For this review, take the finished solid that the model builds, in its own axes (mm). A direction names the side the tool comes from. Round coordinates to 2 decimals unless told otherwise and drop trailing zeros. Order: outer loops, then holes, each group sorted by start corner. A loop starts at its lowest first (then second) coordinate and runs counter-clockwise, first axis right, second up. Notation, with made-up numbers: (35.25, 86) -> (78.25, 86) arc R13 cw to (78.25, 94) -> close; hole circle Ø6 at (85, 14.25). An arc over 180 degrees is marked (long way). Use a Markdown table: item, result. Add a question column.
1) Clearance check with flat-ended pins moving along their axes: P1, Ø3, axis at y = -11.5, z = 10.5, coming from the +X side; P2, Ø3, axis at y = -13.5, z = 4, coming from the +X side; P3, Ø4, axis at y = -14.5, z = 8.5, coming from the -X side; P4, Ø3, axis at x = 6.5, y = -12, coming from the +Z side. State where each tip first meets the part, or that it passes through.
2) Consider section B-B (y = -14.5). Give the number of separate pieces and of enclosed holes in the cut face, plus the area to 3 significant figures.
3) Consider section A-A (z = 7.25). State the section outline as (x, y) points, plus the area to 3 significant figures.
4) Consider section D-D (z = 5). State the section outline as (x, y) points, plus the area to 3 significant figures.
5) Wall thickness on line 1 along X through (y, z) = (-12, 5.5); line 2 along Z through (x, y) = (3.5, -11.25); line 3 along Z through (x, y) = (-2, -15.5): over which ranges is each line inside the solid? List them lowest first. Write a range as [from, to].
6) Draft analysis for pull direction Z (two halves, no side actions). For faces 1 (the face through (4.717, -11, 8)), 2 (the face through (10.95, -12.46, 5.44)), 3 (the face through (2, -11.625, 8)), state which applies: pulls with the +Z half, pulls with the -Z half, needs draft (parallel to the pull), parting line crosses it, or undercut.
7) Consider section C-C (x = 0.25). State the section outline as (y, z) points, plus the area to 3 significant figures.
8) Machinability: for faces 4 (the face through (-3, -12, 6.35)), 5 (the face through (2, -11.625, 11)), 6 (the face through (1.656, -15.016, 11.611)), which of the approach directions +Z, -Z, +X, -X, +Y, -Y give a long, thin tool a straight path to every point of the face, cutting with its end or side? Answer none if there is none.
```python
from build123d import *

# Parameters (mm, degrees)
F0_W        = 20.6375
F0_H        = 7
F1_DEPTH    = 6.35
F2_R        = 2.794
F3_DEPTH    = 8
F4_R        = 3.17499
F5_W        = 6.0368906707
F5_H        = 7
F6_DEPTH    = 6.35
F7_T1_DEPTH = 23.8168906707
F8_W        = 2
F8_H        = 5
F9_DEPTH    = 6.35
F10_W       = 1.5076477192
F10_H       = 2
F10_W_2     = 1.4923522808
F10_W_3     = 2
F10_H_2     = 1.5520717202
F11_DEPTH   = 6.35


# Not quite as in the source:
# - a fillet or chamfer that OpenCascade refuses, or shapes differently, is made with other operations: its cross-section is extruded or revolved along the edge and cut away or added
# - a fillet or chamfer is up to 0.001 mm smaller than in the source, because OpenCascade refuses the exact size


with BuildPart() as f1:
    # F0 (on Top) → F1 (new body)
    with BuildSketch(Plane.XY):
        with Locations((1.5829298645, -12.5110630834)):
            Rectangle(F0_W, F0_H)
    extrude(amount=F1_DEPTH)

    # F2 (on face) → F3 (cut)
    with BuildSketch(Plane.XZ.offset(16.0110630834)):
        with Locations((-5.4325845507, 3.1855095279)):
            Circle(F2_R)
        with Locations((1.5883980845, 3.2361580911)):
            Circle(F2_R)
        with Locations((8.5595190756, 3.1868351264)):
            Circle(F2_R)
    extrude(amount=-F3_DEPTH, mode=Mode.SUBTRACT)

    # F4 (radius 3.175 in the source; OpenCascade refuses exactly that, so slightly less here)
    f4_edges = [f1.edges().sort_by_distance(p)[0] for p in [
        (11.90168, -12.511063, 6.35),
        (11.90168, -12.511063, 0),
        (-8.73582, -12.511063, 6.35),
        (-8.73582, -12.511063, 0),
    ]]
    fillet(f4_edges, radius=F4_R)

    # F5 (on face) → F6 (join)
    with BuildSketch(Plane.XY.offset(6.35)):
        with Locations((1.6981104854, -12.5110630834)):
            Rectangle(F5_W, F5_H)
    extrude(amount=F6_DEPTH)

    # F7: fillet of radius 3.556 on 2 edges, made by hand

    # F7_s2 → F7_t1 (cut)
    with BuildSketch(Plane.YZ.offset(-10.2103348499)):
        with BuildLine():
            ThreePointArc((-16.0110630834, 9.144), (-14.9695347973, 11.6584717139), (-12.4550630834, 12.7))
            Line((-12.4550630834, 12.7), (-16.0110630834, 12.7))
            Line((-16.0110630834, 12.7), (-16.0110630834, 9.144))
        make_face()
        with BuildLine():
            ThreePointArc((-9.0110630834, 9.144), (-10.0525913695, 11.6584717139), (-12.5670630834, 12.7))
            Line((-12.5670630834, 12.7), (-9.0110630834, 12.7))
            Line((-9.0110630834, 12.7), (-9.0110630834, 9.144))
        make_face()
    extrude(amount=F7_T1_DEPTH, mode=Mode.SUBTRACT)

    # F8 (on face) → F9 (cut)
    with BuildSketch(Plane(origin=(-1.3203348499, 0, 0), x_dir=(0, -1, 0), z_dir=(-1, 0, 0))):
        with Locations((12.6245897673, 9.4653457722)):
            Rectangle(F8_W, F8_H)
    extrude(amount=-F9_DEPTH, mode=Mode.SUBTRACT)

    # F10 (on face) → F11 (cut)
    with BuildSketch(Plane.YZ.offset(4.7165558208)):
        with Locations((-14.3784136269, 9.5174174924)):
            Rectangle(F10_W, F10_H)
        with Locations((-10.8784136269, 9.5174174924)):
            Rectangle(F10_W_2, F10_H)
        with Locations((-12.6245897673, 7.7413816323)):
            Rectangle(F10_W_3, F10_H_2)
    extrude(amount=-F11_DEPTH, mode=Mode.SUBTRACT)


solid = f1.part
```
Results list:
| question | item | result |
|---|---|---|
| 1 | P1 | x = 4.72 |
| 1 | P2 | x = 11.9 |
| 1 | P3 | x = -1.32 |
| 1 | P4 | z = 6.35 |
| 2 | separate pieces | 2 |
| 2 | enclosed holes | 3 |
| 2 | area | 71.2 mm2 |
| 3 | outline | (-1.32, -16.01) -> (4.72, -16.01) -> (4.72, -13.62) -> (-1.32, -13.62) -> close; (-1.32, -11.62) -> (4.72, -11.62) -> (4.72, -9.01) -> (-1.32, -9.01) -> close |
| 3 | area | 30.2 mm2 |
| 4 | outline | (-8.16, -16.01) -> (-7.56, -16.01) -> (-7.56, -9.01) -> (-8.16, -9.01) -> close; (-3.31, -16.01) -> (-0.58, -16.01) -> (-0.58, -9.01) -> (-3.31, -9.01) -> close; (3.76, -16.01) -> (6.43, -16.01) -> (6.43, -9.01) -> (3.76, -9.01) -> close; (10.69, -16.01) -> (11.32, -16.01) -> (11.32, -9.01) -> (10.69, -9.01) -> close |
| 4 | area | 46.5 mm2 |
| 5 | line 1 | [-7.72, -7], [-3.87, -0.05], [3.23, 6.99], [10.13, 10.89] |
| 5 | line 2 | [0, 1.2], [5.27, 8.52], [10.52, 12.45] |
| 5 | line 3 | [0, 6.35] |
| 6 | face 1 | needs draft |
| 6 | face 2 | pulls with the +Z half |
| 6 | face 3 | undercut |
| 7 | outline | (-16.01, 0) -> (-9.01, 0) -> (-9.01, 0.78) -> (-16.01, 0.78) -> close; (-16.01, 5.69) -> (-9.01, 5.69) -> (-9.01, 9.14) arc R3.56 ccw to (-12.51, 12.7) arc R3.56 ccw to (-16.01, 9.14) -> close; hole (-15.13, 8.52) -> (-13.62, 8.52) -> (-13.62, 6.97) -> (-11.62, 6.97) -> (-11.62, 8.52) -> (-10.13, 8.52) -> (-10.13, 10.52) -> (-11.62, 10.52) -> (-11.62, 11.97) -> (-13.62, 11.97) -> (-13.62, 10.52) -> (-15.13, 10.52) -> close |
| 7 | area | 33.1 mm2 |
| 8 | face 4 | +Z, -X, +Y, -Y |
| 8 | face 5 | +X, -X |
| 8 | face 6 | +Z, +X, -X, -Y |
